Check sheet for the modelled part. Datum: model origin and axes. Units: mm. Face numbers are marked on the shaded views. A direction names the side the tool comes from. Give positions to 0.01 mm unless a question says otherwise; leave off trailing zeros. Order: outer loops, then holes, each group sorted by start corner. A loop starts at its lowest first (then second) coordinate and runs counter-clockwise, first axis right, second up.
```python
from build123d import *

# Parameters (mm, degrees)
ESQUISSE1_W             = 36.068
ESQUISSE1_H             = 48.26
BOSS_EXTRU_1_DEPTH      = 2
ESQUISSE4_R             = 3
BOSS_EXTRU_2_DEPTH      = 3
ESQUISSE6_R             = 1.45
ENL_V_MAT_EXTRU_1_DEPTH = 31.536569159
ESQUISSE10_W            = 48.26
ESQUISSE10_H            = 2
BOSS_EXTRU_3_DEPTH      = 3
ESQUISSE11_W            = 2.839594579
ESQUISSE11_H            = 48.26
BOSS_EXTRU_4_DEPTH      = 4.6
ESQUISSE12_W            = 48.26
ESQUISSE12_H            = 2.5
BOSS_EXTRU_5_DEPTH      = 5
CONG_1_R                = 10
CONG_2_R                = 10


with BuildPart() as part:
    # Esquisse1 → Boss.-Extru.1 (new body)
    with BuildSketch(Plane(origin=(0, 0, 0), x_dir=(1, 0, 0), z_dir=(0, 1, 0))):
        Rectangle(ESQUISSE1_W, ESQUISSE1_H)
    extrude(amount=BOSS_EXTRU_1_DEPTH)

    # Esquisse4 → Boss.-Extru.2 (add)
    with BuildSketch(Plane(origin=(0, 2, 0), x_dir=(1, 0, 0), z_dir=(0, 1, 0))):
        with Locations(Location((11.3, 18.921, 0), (0, 0, 270))):
            Circle(ESQUISSE4_R)
        with Locations(Location((11.3, -18.925, 0), (0, 0, 270))):
            Circle(ESQUISSE4_R)
    boss_extru_2 = extrude(amount=BOSS_EXTRU_2_DEPTH)

    # Esquisse6 → Enlèv. mat.-Extru.1 (cut, through all)
    with BuildSketch(Plane(origin=(0, 5, 0), x_dir=(1, 0, 0), z_dir=(0, 1, 0))):
        with Locations(Location((11.3, 18.921, 0), (0, 0, 270))):
            Circle(ESQUISSE6_R)
        with Locations(Location((11.3, -18.925, 0), (0, 0, 270))):
            Circle(ESQUISSE6_R)
    enl_v_mat_extru_1 = extrude(amount=-ENL_V_MAT_EXTRU_1_DEPTH, mode=Mode.SUBTRACT)

    # Symétrie1: Boss.-Extru.2, Enlèv. mat.-Extru.1 across plane
    add(boss_extru_2.mirror(Plane(origin=(0, 0, 0), x_dir=(0, 0, 1), z_dir=(1, 0, 0))))
    add(enl_v_mat_extru_1.mirror(Plane(origin=(0, 0, 0), x_dir=(0, 0, 1), z_dir=(1, 0, 0))), mode=Mode.SUBTRACT)

    # Esquisse10 → Boss.-Extru.3 (add)
    with BuildSketch(Plane(origin=(18.034, 0, 0), x_dir=(0, 0, -1), z_dir=(1, 0, 0))):
        with Locations((0, 1)):
            Rectangle(ESQUISSE10_W, ESQUISSE10_H)
    extrude(amount=BOSS_EXTRU_3_DEPTH)

    # Esquisse11 → Boss.-Extru.4 (add)
    with BuildSketch(Plane(origin=(0, 0, 0), x_dir=(-1, 0, 0), z_dir=(0, -1, 0))):
        with Locations((-19.614202711, 0)):
            Rectangle(ESQUISSE11_W, ESQUISSE11_H)
    extrude(amount=BOSS_EXTRU_4_DEPTH)

    # Esquisse12 → Boss.-Extru.5 (add)
    with BuildSketch(Plane.ZY.offset(-18.194405421)):
        with Locations((0, -3.35)):
            Rectangle(ESQUISSE12_W, ESQUISSE12_H)
    extrude(amount=BOSS_EXTRU_5_DEPTH)

    # Congé1
    # the kernel refuses this fillet: 10 mm, written as the material it adds along each edge
    with BuildSketch(Plane(origin=(-11.3, 2, -18.921), x_dir=(0, 0, 1), z_dir=(1, 0, 0))) as cong_1_piece_1_section:
        with BuildLine():
            CenterArc((10.141428429, -10), CONG_1_R, 90, 45.572995999)
            Line((10.141428429, 0), (10.141428429, 0.2))
            Line((10.141428429, 0.2), (3, 0.2))
            Line((3, 0.2), (2.8, 0))
            ThreePointArc((2.8, 0), (2.8, -1.5), (2.857171431, -2.86))
            Line((2.857171431, -2.86), (3, -3))
        make_face()
    cong_1_piece_1 = revolve(axis=Axis((-11.3, 2, -18.921), (0, -1, 0)), mode=Mode.PRIVATE)
    cong_1_piece_1 = split(cong_1_piece_1, bisect_by=Plane(origin=(-14.721075744, 4.069321611, -24.13), z_dir=(0, 0, 1)), keep=Keep.TOP, mode=Mode.PRIVATE)
    cong_1_piece_1 = split(cong_1_piece_1, bisect_by=Plane(origin=(-18.034, 4.069321611, -16.945840998), z_dir=(1, 0, 0)), keep=Keep.TOP, mode=Mode.PRIVATE)
    add(cong_1_piece_1)
    with BuildSketch(Plane(origin=(-11.3, 2, 18.925), x_dir=(0, 0, 1), z_dir=(1, 0, 0))) as cong_1_piece_2_section:
        with BuildLine():
            CenterArc((10.141428429, -10), CONG_1_R, 90, 45.572995999)
            Line((10.141428429, 0), (10.141428429, 0.2))
            Line((10.141428429, 0.2), (3, 0.2))
            Line((3, 0.2), (2.8, 0))
            ThreePointArc((2.8, 0), (2.8, -1.5), (2.857171431, -2.86))
            Line((2.857171431, -2.86), (3, -3))
        make_face()
    cong_1_piece_2 = revolve(axis=Axis((-11.3, 2, 18.925), (0, -1, 0)), mode=Mode.PRIVATE)
    cong_1_piece_2 = split(cong_1_piece_2, bisect_by=Plane(origin=(-11.3, 2.724138959, 24.13), z_dir=(0, 0, -1)), keep=Keep.TOP, mode=Mode.PRIVATE)
    cong_1_piece_2 = split(cong_1_piece_2, bisect_by=Plane(origin=(-18.034, 2.724138959, 12.680212615), z_dir=(1, 0, 0)), keep=Keep.TOP, mode=Mode.PRIVATE)
    add(cong_1_piece_2)

    # Congé2
    # the kernel refuses this fillet: 10 mm, written as the material it adds along each edge
    with BuildSketch(Plane(origin=(11.3, 2, -18.921), x_dir=(0, 0, 1), z_dir=(-1, 0, 0))) as cong_2_piece_1_section:
        with BuildLine():
            CenterArc((10.141428429, 10), CONG_2_R, 224.427004001, 45.572995999)
            Line((10.141428429, 0), (10.141428429, -0.2))
            Line((10.141428429, -0.2), (3, -0.2))
            Line((3, -0.2), (2.8, 0))
            ThreePointArc((2.8, 0), (2.8, 1.5), (2.857171431, 2.86))
            Line((2.857171431, 2.86), (3, 3))
        make_face()
    cong_2_piece_1 = revolve(axis=Axis((11.3, 2, -18.921), (0, 1, 0)), mode=Mode.PRIVATE)
    cong_2_piece_1 = split(cong_2_piece_1, bisect_by=Plane(origin=(14.72056947, 4.068572758, -24.13), z_dir=(0, 0, 1)), keep=Keep.TOP, mode=Mode.PRIVATE)
    cong_2_piece_1 = split(cong_2_piece_1, bisect_by=Plane(origin=(21.034, 4.068572758, -16.946133295), z_dir=(-1, 0, 0)), keep=Keep.TOP, mode=Mode.PRIVATE)
    add(cong_2_piece_1)
    with BuildSketch(Plane(origin=(11.3, 2, 18.925), x_dir=(0, 0, 1), z_dir=(-1, 0, 0))) as cong_2_piece_2_section:
        with BuildLine():
            CenterArc((10.141428429, 10), CONG_2_R, 224.427004001, 45.572995999)
            Line((10.141428429, 0), (10.141428429, -0.2))
            Line((10.141428429, -0.2), (3, -0.2))
            Line((3, -0.2), (2.8, 0))
            ThreePointArc((2.8, 0), (2.8, 1.5), (2.857171431, 2.86))
            Line((2.857171431, 2.86), (3, 3))
        make_face()
    cong_2_piece_2 = revolve(axis=Axis((11.3, 2, 18.925), (0, 1, 0)), mode=Mode.PRIVATE)
    cong_2_piece_2 = split(cong_2_piece_2, bisect_by=Plane(origin=(21.034, 2.723263104, 12.680580548), z_dir=(-1, 0, 0)), keep=Keep.TOP, mode=Mode.PRIVATE)
    cong_2_piece_2 = split(cong_2_piece_2, bisect_by=Plane(origin=(11.3, 2.723263104, 24.13), z_dir=(0, 0, -1)), keep=Keep.TOP, mode=Mode.PRIVATE)
    add(cong_2_piece_2)


solid = part.part
```
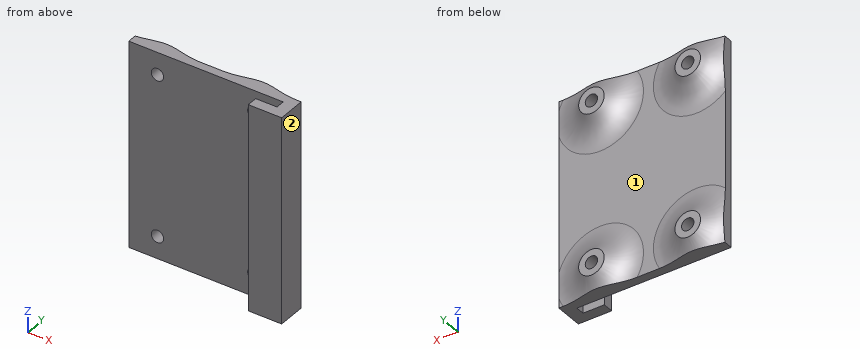
(1) Set-up check for the marked faces 1 and 2: record each of +Z, -Z, +X, -X, +Y, -Y from which the full face is reachable in a straight line by a thin tool's end or side.
Response values:
face 1: +Y
face 2: +Z, -Z, +X, +Y, -Y
(2) Gauge pin test, flat ends, axial feed: pin 1 Ø5 at (x, y) = (2.5, -3) entering from -Z; pin 2 Ø3.5 at (x, z) = (11.3, 18.925) entering from -Y; pin 3 Ø0.8 at (x, z) = (20.5, -23) entering from +Y; pin 4 Ø2 at (y, z) = (-3.5, -9.5) entering from -X. Record the tip position at first contact, or that the pin passes through.
Response values:
pin 1: passes through
pin 2: stops at y = 0
pin 3: stops at y = 2.01
pin 4: stops at x = 13.19
(3) Material ranges on L1, parallel to Z at x = -11.3, y = 1.35 (3 decimals); L2, parallel to X at y = 3.5, z = -19; L3, parallel to Y at x = -16, z = -0.5, recorded low to high.
Response values:
L1: z = -24.13 to -20.371, -17.471 to 17.475, 20.375 to 24.13
L2: x = -16.17 to -12.75, -9.85 to -6.43, 6.43 to 9.85, 12.75 to 16.17
L3: y = 0 to 2
(4) Cross-section at B-B on z = -2.5. Enter the section's corners in (x, y), then the cut area to 3 significant figures.
Response values:
outline: (-18.03, 0) - (18.19, 0) - (18.19, -2.1) - (13.19, -2.1) - (13.19, -4.6) - (21.03, -4.6) - (21.03, 2) - (-18.03, 2) - close
area: 104 mm2
(5) Cross-section at C-C on x = 0. Enter the section's corners in (y, z), then the cut area to 3 significant figures.
Response values:
outline: (0, -24.13) - (2, -24.13) - (2, 24.13) - (0, 24.13) - close
area: 96.5 mm2
(6) Cross-section at A-A on x = -11.3. Enter the section's corners in (y, z) (3 decimals), then the cut area to 3 significant figures.
Response values:
outline: (0, -24.13) - (3.301, -24.13) arc R10 cw to (5, -21.921) - (5, -20.371) - (0, -20.371) - close; (0, -17.471) - (5, -17.471) - (5, -15.921) arc R10 cw to (2, -8.78) - (2, 8.784) arc R10 cw to (5, 15.925) - (5, 17.475) - (0, 17.475) - close; (0, 20.375) - (5, 20.375) - (5, 21.925) arc R10 cw to (3.303, 24.13) - (0, 24.13) - close
area: 126 mm2
